Geometry check sheet. Reference: the model listing, model coordinates, mm. A direction names the side the tool comes from. Coordinates: 2 decimals unless noted, no trailing zeros. Write each loop counter-clockwise with the first axis right and the second up, starting at its lowest first coordinate (ties: lowest second). Pieces come first, ordered by that corner, then holes. Notation, with made-up numbers: (32.25, 63.5) -> (88.25, 63.5) arc R28 cw to (88.25, 94.5) -> close; hole circle Ø6 at (-8, -9). An arc over 180 degrees is marked (long way). Put each result on its own line as item: value. Start each with the question number.
from build123d import *

# Parameters (mm, degrees)
SKETCH1_W           = 101.6
SKETCH1_H           = 88.9
BOSS_EXTRUDE1_DEPTH = 17.78
SKETCH2_R           = 3.175
CUT_EXTRUDE1_DEPTH  = 18.78
FILLET1_R           = 31.75
SKETCH3_W           = 38.1
SKETCH3_H           = 38.1
CUT_EXTRUDE2_DEPTH  = 18.78


with BuildPart() as part:
    # Sketch1 → Boss-Extrude1 (new body)
    with BuildSketch(Plane.XY):
        with Locations((4.927530561, 7.6106367)):
            Rectangle(SKETCH1_W, SKETCH1_H)
    extrude(amount=BOSS_EXTRUDE1_DEPTH)

    # Sketch2 → Cut-Extrude1 (cut, through all)
    with BuildSketch(Plane.XY.offset(17.78)):
        with Locations((-20.472469439, -11.4393633)):
            Circle(SKETCH2_R)
        with Locations((30.327530561, -11.4393633)):
            Circle(SKETCH2_R)
    extrude(amount=-CUT_EXTRUDE1_DEPTH, mode=Mode.SUBTRACT)

    # Fillet1
    fillet1_edges = [part.edges().sort_by_distance(p)[0] for p in [
        (-45.872469439, 52.0606367, 8.89),
        (55.727530561, 52.0606367, 8.89),
    ]]
    fillet(fillet1_edges, radius=FILLET1_R)

    # Sketch3 → Cut-Extrude2 (cut, through all)
    with BuildSketch(Plane.XY.offset(17.78)):
        with Locations((4.927530561, 33.0106367)):
            Rectangle(SKETCH3_W, SKETCH3_H)
    extrude(amount=-CUT_EXTRUDE2_DEPTH, mode=Mode.SUBTRACT)


solid = part.part
Item 1: Section check B-B, the plane z = 10. Enter the section's corners in (x, y) (3 decimals).
Item 2: Scan lines: line 1 along X through (y, z) = (-11, 6.5); line 2 along X through (y, z) = (20.5, 8.5); line 3 along Y through (x, z) = (23, 1). Record each from-to range of solid material in increasing order. Write a range as [from, to].
Item 3: Go/stop test with flat-tipped pins: P1, Ø10, axis at x = 41.5, z = 15.5, coming from the +Y side; P2, Ø9, axis at x = 0, z = 9.5, coming from the +Y side. Record where each tip stops, or that it passes through.
Item 4: Section check D-D, the plane x = 35.5. Enter the section's corners in (y, z), and give its area (3 significant figures).
Item 5: Access from +Z, -Z, +X, -X, +Y, -Y to the whole of each face (thin tool, end or side, straight path). Record for faces 1 (the cylindrical face through (27.808, -13.371, 9.014)), 2 (the flat face through (23.978, 33, 9)).
Item 6: Section check C-C, the plane x = -6. Enter the section's corners in (y, z).
Item 7: Mould release check, pull along X, two halves, no side actions. Record for faces 3 (the flat face through (-14.122, 33, 9)), 4 (the flat face through (-45.872, -9, 9)), 5 (the flat face through (4, -2, 17.78)): released by +X, released by -X, zero draft, split by the parting line, or undercut.
Item 8: Section check A-A, the plane y = 32.5. Enter the section's corners in (x, z), and give its area (3 significant figures).
From the geometry:
1. outline: (-45.872, -36.839) -> (55.728, -36.839) -> (55.728, 20.311) arc R31.75 ccw to (23.978, 52.061) -> (23.978, 13.961) -> (-14.122, 13.961) -> (-14.122, 52.061) arc R31.75 ccw to (-45.872, 20.311) -> close; hole circle Ø6.35 at (-20.472, -11.439); hole circle Ø6.35 at (30.328, -11.439)
2. line 1: [-45.87, -23.62], [-17.33, 27.18], [33.47, 55.73]
2. line 2: [-45.87, -14.12], [23.98, 55.73]
2. line 3: [-36.84, 13.96]
3. P1: y = 49.49
3. P2: y = 13.96
4. outline: (-36.84, 0) -> (49.9, 0) -> (49.9, 17.78) -> (-36.84, 17.78) -> close
4. area: 1,540 mm²
5. face 1: +Z, -Z
5. face 2: +Z, -Z, +Y
6. outline: (-36.84, 0) -> (13.96, 0) -> (13.96, 17.78) -> (-36.84, 17.78) -> close
7. face 3: undercut
7. face 4: released by -X
7. face 5: zero draft
8. outline: (-43.44, 0) -> (-14.12, 0) -> (-14.12, 17.78) -> (-43.44, 17.78) -> close; (23.98, 0) -> (53.29, 0) -> (53.29, 17.78) -> (23.98, 17.78) -> close
8. area: 1,040 mm²
